Source: CAD feature listing. Evaluate the final solid. Frame: model axes, mm. Coordinates: 2 decimals unless noted, no trailing zeros. Write each loop counter-clockwise with the first axis right and the second up, starting at its lowest first coordinate (ties: lowest second). Pieces come first, ordered by that corner, then holes. Notation, with made-up numbers: (-11.75, 80.25) - (7.25, 80.25) arc R21 cw to (7.25, 108.25) - close; hole circle Ø10 at (17.5, 0.5). An arc over 180 degrees is marked (long way). One line per question, with ' | ' between items.
from build123d import *

# Parameters (mm, degrees)
F1_DEPTH = 25.4


# Not quite as in the source:
# - the program builds the solid bodies; features that only make, move or delete a surface that nothing else refers to are left out


with BuildPart() as f1:
    # F0 (on Front) → F1 (new body)
    with BuildSketch(Plane.XZ):
        with BuildLine():
            ThreePointArc((-11.1825731718, -0.6491680963), (-7.9102714826, -7.9308869007), (-0.6200603199, -11.1842249244))
            Line((-0.6200603199, -11.1842249244), (-0.6200603199, -10.9043848611))
            ThreePointArc((-0.6200603199, -10.9043848611), (-7.7127048151, -7.7333219534), (-10.902690713, -0.6491680963))
            Line((-10.902690713, -0.6491680963), (-11.1825731718, -0.6491680963))
        make_face()
        with BuildLine():
            Line((-10.902690713, 0.6491680963), (-11.1825731718, 0.6491680963))
            Line((-11.1825731718, 0.6491680963), (-11.1825731718, -0.6491680963))
            Line((-11.1825731718, -0.6491680963), (-10.902690713, -0.6491680963))
            ThreePointArc((-10.902690713, -0.6491680963), (-10.922, 0), (-10.902690713, 0.6491680963))
        make_face()
        with BuildLine():
            Line((-0.6200603199, 10.9043848611), (-0.6200603199, 11.1842249244))
            ThreePointArc((-0.6200603199, 11.1842249244), (-7.9102714826, 7.9308869007), (-11.1825731718, 0.6491680963))
            Line((-11.1825731718, 0.6491680963), (-10.902690713, 0.6491680963))
            ThreePointArc((-10.902690713, 0.6491680963), (-7.7127048151, 7.7333219534), (-0.6200603199, 10.9043848611))
        make_face()
        with BuildLine():
            Line((0.6200603199, 10.9043848611), (0.6200603199, 11.1842249244))
            Line((0.6200603199, 11.1842249244), (-0.6200603199, 11.1842249244))
            Line((-0.6200603199, 11.1842249244), (-0.6200603199, 10.9043848611))
            ThreePointArc((-0.6200603199, 10.9043848611), (0, 10.922), (0.6200603199, 10.9043848611))
        make_face()
        with BuildLine():
            Line((10.902690713, 0.6491680963), (11.1825731718, 0.6491680963))
            ThreePointArc((11.1825731718, 0.6491680963), (7.9102714826, 7.9308869007), (0.6200603199, 11.1842249244))
            Line((0.6200603199, 11.1842249244), (0.6200603199, 10.9043848611))
            ThreePointArc((0.6200603199, 10.9043848611), (7.7127048151, 7.7333219534), (10.902690713, 0.6491680963))
        make_face()
        with BuildLine():
            Line((11.1825731718, -0.6491680963), (11.1825731718, 0.6491680963))
            Line((11.1825731718, 0.6491680963), (10.902690713, 0.6491680963))
            ThreePointArc((10.902690713, 0.6491680963), (10.917171611, 0.3247276035), (10.922, 0))
            ThreePointArc((10.922, 0), (10.917171611, -0.3247276035), (10.902690713, -0.6491680963))
            Line((10.902690713, -0.6491680963), (11.1825731718, -0.6491680963))
        make_face()
        with BuildLine():
            ThreePointArc((0.6200603199, -11.1842249244), (7.9102714826, -7.9308869007), (11.1825731718, -0.6491680963))
            Line((11.1825731718, -0.6491680963), (10.902690713, -0.6491680963))
            ThreePointArc((10.902690713, -0.6491680963), (7.7127048151, -7.7333219534), (0.6200603199, -10.9043848611))
            Line((0.6200603199, -10.9043848611), (0.6200603199, -11.1842249244))
        make_face()
        with BuildLine():
            Line((-0.6200603199, -11.1842249244), (0.6200603199, -11.1842249244))
            Line((0.6200603199, -11.1842249244), (0.6200603199, -10.9043848611))
            ThreePointArc((0.6200603199, -10.9043848611), (0, -10.922), (-0.6200603199, -10.9043848611))
            Line((-0.6200603199, -10.9043848611), (-0.6200603199, -11.1842249244))
        make_face()
    extrude(amount=F1_DEPTH)


solid = f1.part
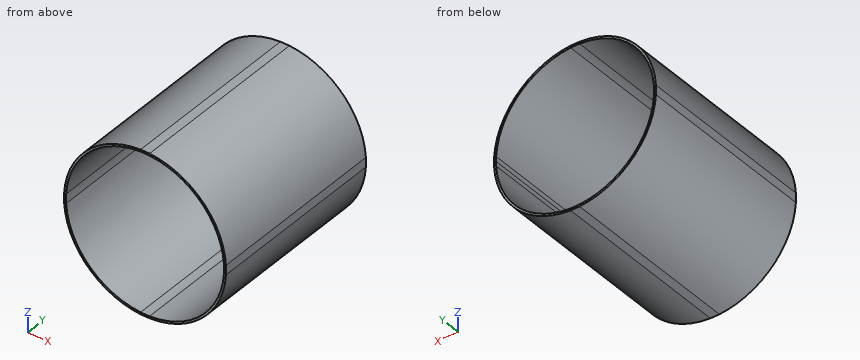
Item 1: Cut plane B-B on y = -13.5. Return loops of the section in (x, z).
Check sheet entries:
outline: (-11.18, -0.65) arc R11.2 ccw to (-0.62, -11.18) - (0.62, -11.18) arc R11.2 ccw to (11.18, -0.65) - (11.18, 0.65) arc R11.2 ccw to (0.62, 11.18) - (-0.62, 11.18) arc R11.2 ccw to (-11.18, 0.65) - close; hole circle Ø21.84 at (0, 0)
Item 2: Cut plane C-C on z = -8. Return loops of the section in (x, y), and give its area (3 significant figures).
Check sheet entries:
outline: (-7.84, -25.4) - (-7.44, -25.4) - (-7.44, 0) - (-7.84, 0) - close; (7.44, -25.4) - (7.84, -25.4) - (7.84, 0) - (7.44, 0) - close | area: 20.6 mm²
Item 3: Ray query, line 1 along Z through (x, y) = (6.25, -11.25); line 2 along X through (y, z) = (-7, -2.75); line 3 along Z through (x, y) = (5, -22.25). Return the intervals inside material, ascending. Write a range as [from, to].
Check sheet entries:
line 1: [-9.3, -8.96], [8.96, 9.3] | line 2: [-10.86, -10.57], [10.57, 10.86] | line 3: [-10.02, -9.71], [9.71, 10.02]
Item 4: Pin query (flat end, axial travel): pin 1 Ø2 at (x, z) = (-8.5, 6.5) entering from +Y; pin 2 Ø3 at (y, z) = (-13, -8) entering from +X; pin 3 Ø10 at (x, y) = (8, -9.5) entering from -Z. Return the tip coordinate at first contact, or that it passes through.
Check sheet entries:
pin 1: y = 0 | pin 2: x = 9.12 | pin 3: z = -10.79
Item 5: Cut plane A-A on x = 0. Return loops of the section in (y, z).
Check sheet entries:
outline: (-25.4, -11.18) - (0, -11.18) - (0, -10.92) - (-25.4, -10.92) - close; (-25.4, 10.92) - (0, 10.92) - (0, 11.18) - (-25.4, 11.18) - close
